Source: three-view drawing plus pictorial views. Frame: mm from the lowest corner of the part. A direction names the side the tool comes from. Coordinates: 2 decimals unless noted, no trailing zeros. Order: outer loops, then holes, each group sorted by start corner. A loop starts at its lowest first (then second) coordinate and runs counter-clockwise, first axis right, second up. Notation, with made-up numbers: M 51,-5 L 83,-5 A20 cw 83,29 Z; hole C 16.25,-9 d2. An arc over 180 degrees is marked long. Use CSV: the item, a comma, the result in double quotes. Start each with the question number.
Q1. First-contact query: P1, Ø3.5, axis at x = 64.5, z = 24.5, coming from the -Y side; P2, Ø9.5, axis at x = 34.5, z = 28.5, coming from the +Y side; P3, Ø3.5, axis at x = 33.5, y = 45, coming from the +Z side. Flat tips, straight axial feed; report the tip coordinate or a pass-through.
Q2. Section query D-D, the plane x = 37.5. Output: boundary loops of the cut face in (y, z).
Q3. Access query for the marked faces 1, 2, 3, 4 and 5. Directions: +Z, -Z, +X, -X, +Y, -Y. A direction counts if a zero-diameter tool reaches every point of the face in a straight line with its end or side. Return the directions, or none.
Q4. Section query B-B, the plane y = 28. Output: boundary loops of the cut face in (x, z).
Q5. Section query C-C, the plane y = 12. Output: boundary loops of the cut face in (x, z).
Q6. Mould query, pull axis Z, two halves, no side actions, for the marked faces 6, 7 and 8. Classes: +Z half, -Z half, draft (parallel to the pull), parting line (faces both ways), or undercut.
Q7. Ray query, probe 1 along X at (y, z) = (43, 7); probe 2 along X at (y, z) = (6.5, 31); probe 3 along X at (y, z) = (24.5, 3.5). Return the intervals inside material, ascending.
Q8. Section query A-A, the plane z = 7.5. Output: boundary loops of the cut face in (x, y).
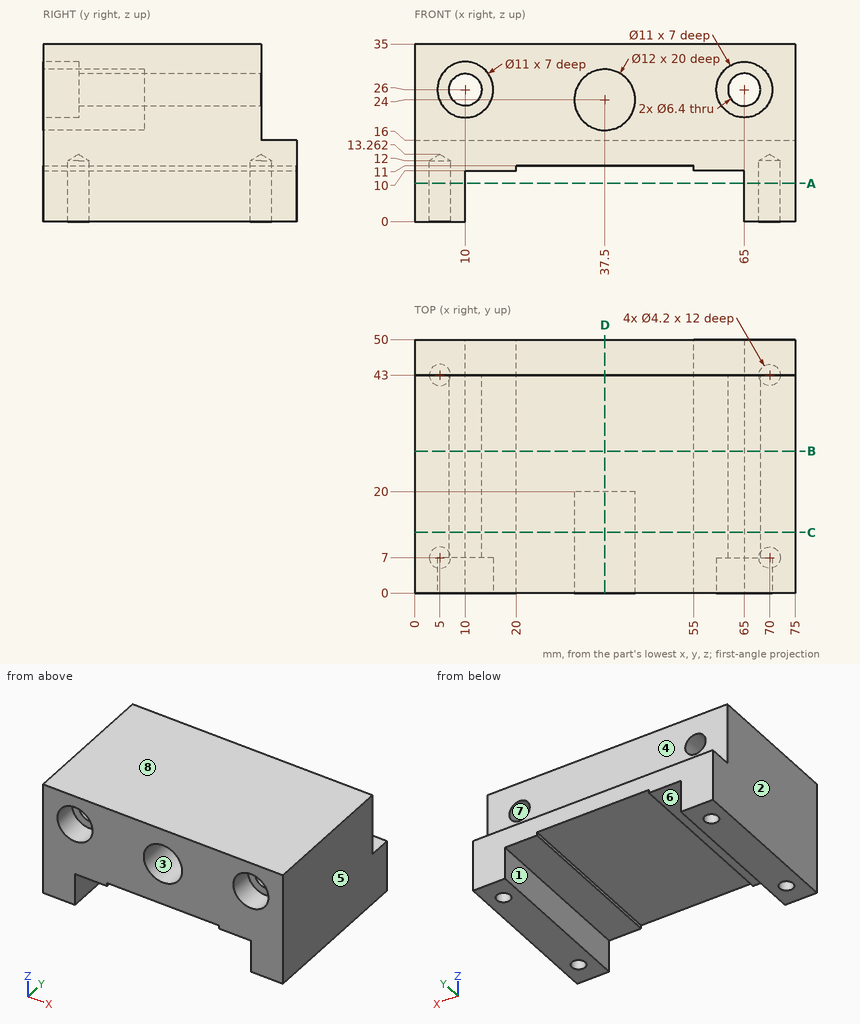
Responses:
1,P1,"stops at y = 7"
1,P2,"stops at y = 43"
1,P3,"stops at z = 16"
2,outline,"M 0,11 L 50,11 L 50,16 L 43,16 L 43,35 L 0,35 L 0,30 L 20,30 L 20,18 L 0,18 Z"
3,face 1,"-Z, +Y, -Y"
3,face 2,"+Z, -Z, -X, +Y, -Y"
3,face 3,"-Y"
3,face 4,"+Z, +X, -X, +Y"
3,face 5,"+Z, -Z, +X, +Y, -Y"
4,outline,"M 0,0 L 10,0 L 10,10 L 20,10 L 20,11 L 55,11 L 55,10 L 65,10 L 65,0 L 75,0 L 75,35 L 0,35 Z; hole C 10,26 d6.4; hole C 65,26 d6.4"
5,outline,"M 0,0 L 10,0 L 10,10 L 20,10 L 20,11 L 55,11 L 55,10 L 65,10 L 65,0 L 75,0 L 75,35 L 0,35 Z; hole C 10,26 d6.4; hole C 37.5,24 d12; hole C 65,26 d6.4"
6,face 6,"-Z half"
6,face 7,"undercut"
6,face 8,"+Z half"
7,probe 1,"x = 0 to 2.9, 7.1 to 10, 65 to 67.9, 72.1 to 75"
7,probe 2,"x = 0 to 7.71, 12.29 to 62.71, 67.29 to 75"
7,probe 3,"x = 0 to 10, 65 to 75"
8,outline,"M 0,0 L 10,0 L 10,50 L 0,50 Z; M 65,0 L 75,0 L 75,50 L 65,50 Z; hole C 5,7 d4.2; hole C 5,43 d4.2; hole C 70,7 d4.2; hole C 70,43 d4.2"
